from build123d import *

# Parameters (mm, degrees)
F0_W     = 2.5
F0_H     = 3
F1_DEPTH = 500
F2_R     = 2
F3_R     = 7
F3_R_2   = 7.5
F4_DEPTH = 8


with BuildPart() as f1:
    # F0 (on Top) → F1 (new body)
    with BuildSketch(Plane.XY):
        with BuildLine():
            Line((-20.5, 17), (-20.5, -20.5))
            Line((-20.5, -20.5), (20.5, -20.5))
            Line((20.5, -20.5), (20.5, 17))
            ThreePointArc((20.5, 17), (17, 20.5), (13.5, 17))
            Line((13.5, 17), (13.5, 14))
            Line((13.5, 14), (16, 14))
            Line((16, 14), (16, 17))
            ThreePointArc((16, 17), (17, 18), (18, 17))
            Line((18, 17), (18, -18))
            Line((18, -18), (-18, -18))
            Line((-18, -18), (-18, 17))
            ThreePointArc((-18, 17), (-17, 18), (-16, 17))
            Line((-16, 17), (-13.5, 17))
            ThreePointArc((-13.5, 17), (-17, 20.5), (-20.5, 17))
        make_face()
        with Locations((-14.75, 15.5)):
            Rectangle(F0_W, F0_H)
    extrude(amount=F1_DEPTH)

    # F2
    f2_edges = [f1.edges().sort_by_distance(p)[0] for p in [
        (-20.5, -20.5, 250),
        (20.5, -20.5, 250),
        (-18, -18, 250),
        (18, -18, 250),
    ]]
    fillet(f2_edges, radius=F2_R)

    # F3 (on face) → F4 (join)
    with BuildSketch(Plane(origin=(0, 0, 0), x_dir=(1, 0, 0), z_dir=(0, 0, -1))):
        with BuildLine():
            Line((17.5, 66.5), (-17.5, 66.5))
            ThreePointArc((-17.5, 66.5), (-21.035534, 65.035534), (-22.5, 61.5))
            Line((-22.5, 61.5), (-22.5, -61.5))
            ThreePointArc((-22.5, -61.5), (-21.035534, -65.035534), (-17.5, -66.5))
            Line((-17.5, -66.5), (17.5, -66.5))
            ThreePointArc((17.5, -66.5), (21.035534, -65.035534), (22.5, -61.5))
            Line((22.5, -61.5), (22.5, 61.5))
            ThreePointArc((22.5, 61.5), (21.035534, 65.035534), (17.5, 66.5))
        make_face()
        with Locations((0, -52)):
            Circle(F3_R, mode=Mode.SUBTRACT)
        with Locations((0, 45)):
            Circle(F3_R_2, mode=Mode.SUBTRACT)
    extrude(amount=F4_DEPTH)


solid = f1.part
Verification items for the finished model (mm, model axes). A direction names the side the tool comes from. Coordinates: 2 decimals unless noted, no trailing zeros. Loops run counter-clockwise (first coordinate to the right, second up) from the corner with the lowest first, then second, coordinate; pieces in that order, holes last. Notation, with made-up numbers: (43, 18.5) -> (68, 18.5) arc R23 cw to (68, 51.5) -> close; hole circle Ø11 at (-16.5, 37). An arc over 180 degrees is marked (long way). Write each question's results on one line, items separated by ' | '.
Item 1: Section check A-A, the plane y = 52. Enter the section's corners in (x, z), plus the area to 3 significant figures.
Found:
outline: (-22.5, -8) -> (-7, -8) -> (-7, 0) -> (-22.5, 0) -> close; (7, -8) -> (22.5, -8) -> (22.5, 0) -> (7, 0) -> close | area: 248 mm2
Item 2: Section check D-D, the plane y = 9. Enter the section's corners in (x, z).
Found:
outline: (-22.5, -8) -> (22.5, -8) -> (22.5, 0) -> (20.5, 0) -> (20.5, 500) -> (18, 500) -> (18, 0) -> (-18, 0) -> (-18, 500) -> (-20.5, 500) -> (-20.5, 0) -> (-22.5, 0) -> close
Item 3: Tool access check on faces 1 (the face through (-20.5, -1, 246)), 2 (the face through (0, -20.5, 246)), 3 (the face through (20.5, -1, 246)), 4 (the face through (-18, 0, 246)). Record the directions out of +Z, -Z, +X, -X, +Y, -Y that give a thin tool (end or side, any length) a straight path to the whole face; none if there is none.
Found:
face 1: +Z, -X, +Y, -Y | face 2: +Z, +X, -X, -Y | face 3: +Z, +X, +Y, -Y | face 4: +Z
Item 4: Section check C-C, the plane z = 187.5. Enter the section's corners in (x, y), plus the area to 3 significant figures.
Found:
outline: (-20.5, -18.5) arc R2 ccw to (-18.5, -20.5) -> (18.5, -20.5) arc R2 ccw to (20.5, -18.5) -> (20.5, 17) arc R3.5 ccw to (13.5, 17) -> (13.5, 14) -> (16, 14) -> (16, 17) arc R1 cw to (18, 17) -> (18, -16) arc R2 cw to (16, -18) -> (-16, -18) arc R2 cw to (-18, -16) -> (-18, 17) arc R1 cw to (-16, 17) -> (-16, 14) -> (-13.5, 14) -> (-13.5, 17) arc R3.5 ccw to (-20.5, 17) -> close | area: 328 mm2
Item 5: Material ranges on L1, parallel to Y at x = 0, z = -3.25; L2, parallel to X at y = 10, z = 173; L3, parallel to X at y = 52, z = -5, recorded low to high.
Found:
L1: y = -66.5 to -52.5, -37.5 to 45, 59 to 66.5 | L2: x = -20.5 to -18, 18 to 20.5 | L3: x = -22.5 to -7, 7 to 22.5
Item 6: Mould release check, pull along X, two halves, no side actions. Record for faces 5 (the face through (-0.91, 45.06, -3.94)), 6 (the face through (0, 66.5, -4)), 7 (the face through (-22.5, -1, -4)): +X half, -X half, draft (parallel to the pull), parting line (faces both ways), or undercut.
Found:
face 5: undercut | face 6: draft | face 7: -X half
Item 7: Gauge pin test, flat ends, axial feed: pin 1 (3.5 mm diameter, centred on y = 16, z = 212, fed in from +X); pin 2 (1.5 mm diameter, centred on x = -14.5, z = 400.5, fed in from +Y); pin 3 (22.5 mm diameter, centred on x = -8, y = 31.5, fed in from +Z). Record the tip position at first contact, or that the pin passes through.
Found:
pin 1: stops at x = 20.5 | pin 2: stops at y = 20.03 | pin 3: stops at z = 0
Item 8: Section check B-B, the plane x = 0. Enter the section's corners in (y, z), plus the area to 3 significant figures.
Found:
outline: (-66.5, -8) -> (-52.5, -8) -> (-52.5, 0) -> (-66.5, 0) -> close; (-37.5, -8) -> (45, -8) -> (45, 0) -> (-18, 0) -> (-18, 500) -> (-20.5, 500) -> (-20.5, 0) -> (-37.5, 0) -> close; (59, -8) -> (66.5, -8) -> (66.5, 0) -> (59, 0) -> close | area: 2,080 mm2
